Geometry check sheet. Reference: drawing and pictorial views, mm from the part's lowest x, y, z. A direction names the side the tool comes from. Give positions to 0.01 mm unless a question says otherwise; leave off trailing zeros. Write each loop counter-clockwise with the first axis right and the second up, starting at its lowest first coordinate (ties: lowest second). Pieces come first, ordered by that corner, then holes.
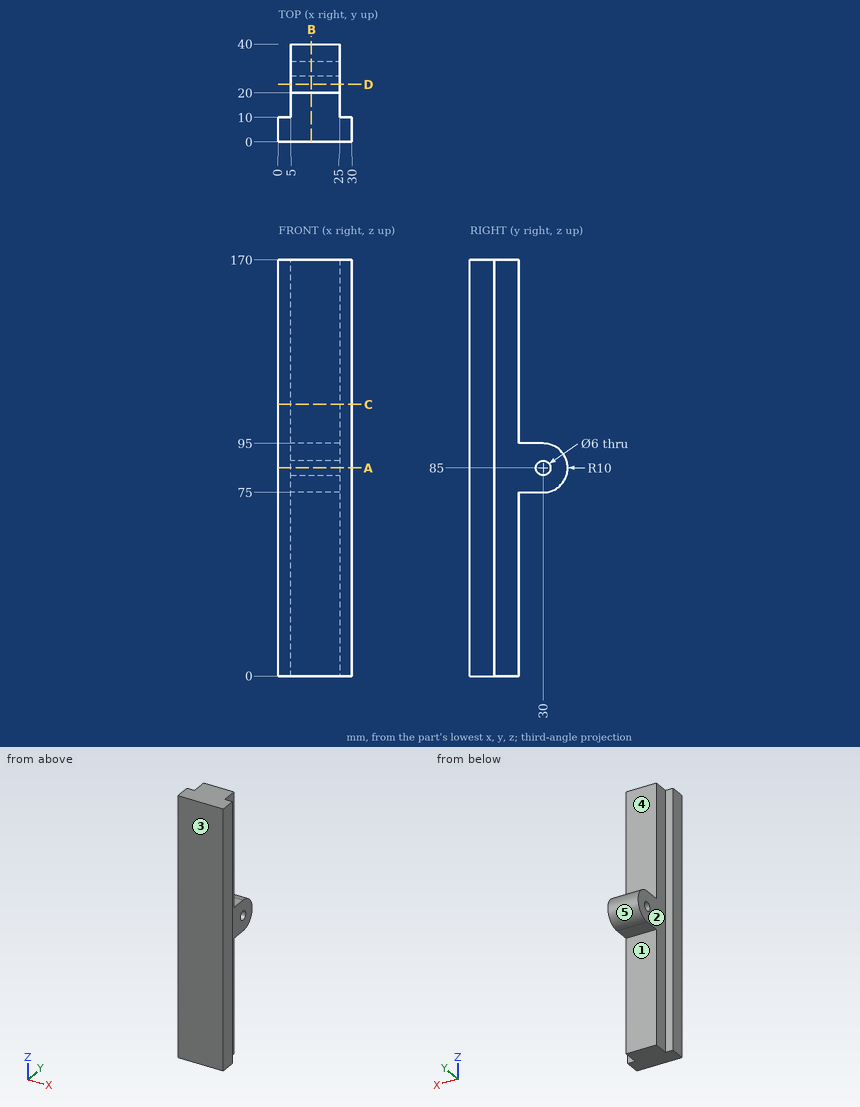
Item 1: Sectioned sample at A-A on z = 85. Record the cut outline in (x, y), then the cut area to 3 significant figures.
Answer key:
outline: (0, 0) - (30, 0) - (30, 10) - (25, 10) - (25, 27) - (5, 27) - (5, 10) - (0, 10) - close; (5, 33) - (25, 33) - (25, 40) - (5, 40) - close
area: 780 mm2
Item 2: Scan lines: line 1 along Y through (x, z) = (18.5, 85); line 2 along Y through (x, z) = (26.25, 147); line 3 along Y through (x, z) = (17, 139.5). Record each from-to range of solid material in increasing order.
Answer key:
line 1: y = 0 to 27, 33 to 40
line 2: y = 0 to 10
line 3: y = 0 to 20
Item 3: Sectioned sample at D-D on y = 23.5. Record the cut outline in (x, z), then the cut area to 3 significant figures.
Answer key:
outline: (5, 75) - (25, 75) - (25, 95) - (5, 95) - close
area: 400 mm2
Item 4: Set-up check for the marked faces 1, 2, 3, 4 and 5: record each of +Z, -Z, +X, -X, +Y, -Y from which the full face is reachable in a straight line by a thin tool's end or side.
Answer key:
face 1: -Z, +X, -X, +Y
face 2: +Z, -Z, -X, +Y
face 3: +Z, -Z, +X, -X, -Y
face 4: +Z, +X, -X, +Y
face 5: +X, -X, +Y
Item 5: Depth check by flat-ended pin: pin 1 (1 mm diameter, centred on x = 22.5, z = 78, fed in from +Y); pin 2 (1.5 mm diameter, centred on x = 3.5, z = 93, fed in from +Y); pin 3 (8 mm diameter, centred on x = 12.5, z = 21, fed in from +Y). Enter the tip coordinate at first touch or a pass-through.
Answer key:
pin 1: stops at y = 37.6
pin 2: stops at y = 10
pin 3: stops at y = 20
Item 6: Sectioned sample at C-C on z = 111. Record the cut outline in (x, y), then the cut area to 3 significant figures.
Answer key:
outline: (0, 0) - (30, 0) - (30, 10) - (25, 10) - (25, 20) - (5, 20) - (5, 10) - (0, 10) - close
area: 500 mm2
Item 7: Sectioned sample at B-B on x = 13.5. Record the cut outline in (y, z), then the cut area to 3 significant figures.
Answer key:
outline: (0, 0) - (20, 0) - (20, 75) - (30, 75) arc R10 ccw to (30, 95) - (20, 95) - (20, 170) - (0, 170) - close; hole circle Ø6 at (30, 85)
area: 3,730 mm2
